Check sheet for the modelled part. Datum: model origin and axes. Units: mm. Face numbers are marked on the shaded views. A direction names the side the tool comes from. Round coordinates to 2 decimals unless told otherwise and drop trailing zeros. Order: outer loops, then holes, each group sorted by start corner. A loop starts at its lowest first (then second) coordinate and runs counter-clockwise, first axis right, second up. Notation, with made-up numbers: (66.25, 49) -> (107.25, 49) arc R21 ccw to (107.25, 72) -> close; hole circle Ø3 at (64.25, 88.25). An arc over 180 degrees is marked (long way). Answer in a Markdown table with one row per item.
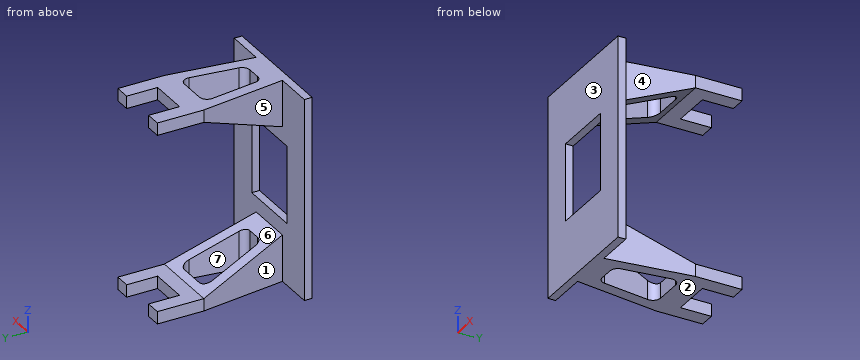
Autodesk Fusion 360 part; units mm, degrees
sketch "Esquisse1" plane through (0, 0, 0) normal (0, 0, 1) x (1, 0, 0)
  line L0 (27.5, 70) -> (52.5, 70)
  line L1 (52.5, 70) -> (52.5, 90)
  line L2 (27.5, 70) -> (27.5, 90)
  line L3 (27.5, 90) -> (17.5, 90)
  line L4 (52.5, 90) -> (62.5, 90)
  line L5 (62.5, 90) -> (62.5, 60)
  line L6 (17.5, 90) -> (17.5, 60)
  line L7 (17.5, 60) -> (25, 5)
  line L8 (25, 5) -> (0, 5)
  line L9 (0, 5) -> (0, 0)
  line L10 (0, 0) -> (80, 0)
  line L11 (80, 0) -> (80, 5)
  line L12 (80, 5) -> (55, 5)
  line L13 (55, 5) -> (62.5, 60)
  dimension "d1" = 70
  dimension "d2" = 25
  dimension "d3" = 20
  dimension "d4" = 10
  dimension "d5" = 30
  dimension "d8" = 5
  dimension "d10" = 10
  dimension "d27" = 80
  dimension "d28" = 45
  dimension "d29" = 17.5
  dimension "d30" = 30
extrude "Extrusion1" add sketch "Esquisse1" along normal blind 130
sketch "Esquisse2" plane through (62.5, 0, 0) normal (1, 0, 0) x (0, 0, -1)
  line L0 (0, 60) -> (0, 90)
  line L1 (0, 90) -> (-130, 90)
  line L2 (-130, 90) -> (-130, 60)
  line L3 (-130, 60) -> (0, 60)
  line L4 (-65, 90) -> (-65, -26) construction
  line L5 (-122, 90) -> (-122, 60)
  line L6 (-122, 60) -> (-100, 5)
  line L7 (-8, 90) -> (-8, 60)
  line L8 (-8, 60) -> (-30, 5)
  line L9 (-100, 5) -> (-30, 5)
  point P0 (-130, 5)
  point P1 (0, 5)
  dimension "d13" = 8
  dimension "d14" = 30
  dimension "d15" = 30
  dimension "d16" = 8
extrude "Extrusion2" cut sketch "Esquisse2" against normal blind 60 contours L3 L6 L8 L9 | L1 L3 L5 L7
sketch "Esquisse3" plane through (0, 0, 130) normal (0, 0, 1) x (1, 0, 0)
  line L0 (27.5, 70) -> (27.5, 90)
  line L1 (27.5, 90) -> (17.5, 90)
  line L2 (17.5, 90) -> (17.5, 60)
  line L3 (17.5, 60) -> (25, 5)
  line L4 (25, 5) -> (0, 5)
  line L5 (0, 5) -> (0, 0)
  line L6 (0, 0) -> (80, 0)
  line L7 (80, 0) -> (80, 5)
  line L8 (80, 5) -> (55, 5)
  line L9 (55, 5) -> (62.5, 60)
  line L10 (62.5, 60) -> (62.5, 90)
  line L11 (62.5, 90) -> (52.5, 90)
  line L12 (52.5, 90) -> (52.5, 70)
  line L13 (52.5, 70) -> (27.5, 70)
  line L14 (26.5252, 49.3244) -> (30.6161, 19.3244)
  line L15 (35.5702, 15) -> (44.4298, 15)
  line L16 (49.3839, 19.3244) -> (53.4748, 49.3244)
  line L17 (48.5207, 55) -> (31.4793, 55)
  arc A0 (31.4793, 55) -> (26.5252, 49.3244) centre (31.4793, 50) ccw
  arc A1 (53.4748, 49.3244) -> (48.5207, 55) centre (48.5207, 50) ccw
  arc A2 (30.6161, 19.3244) -> (35.5702, 15) centre (35.5702, 20) ccw
  arc A3 (44.4298, 15) -> (49.3839, 19.3244) centre (44.4298, 20) ccw
  dimension "d19" = 15
  dimension "d20" = 15
  dimension "d21" = 7.5
  dimension "d22" = 7.5
  dimension "d25" = 5
extrude "Extrusion3" cut sketch "Esquisse3" against normal blind 150 contours L14 L15 L16 L17 A0 A1 A2 A3
sketch "Esquisse4" plane through (0, 5, 0) normal (0, 1, 0) x (-1, 0, 0)
  line L0 (-55, 100) -> (-55, 130)
  line L1 (-55, 130) -> (-80, 130)
  line L2 (-80, 130) -> (-80, 0)
  line L3 (-80, 0) -> (-55, 0)
  line L4 (-55, 0) -> (-55, 30)
  line L5 (-55, 30) -> (-25, 30)
  line L6 (-25, 30) -> (-25, 0)
  line L7 (-25, 0) -> (0, 0)
  line L8 (0, 0) -> (0, 130)
  line L9 (0, 130) -> (-25, 130)
  line L10 (-25, 130) -> (-25, 100)
  line L11 (-25, 100) -> (-55, 100)
  line L12 (-60, 90) -> (-20, 90)
  line L13 (-20, 90) -> (-20, 40)
  line L14 (-20, 40) -> (-60, 40)
  line L15 (-60, 40) -> (-60, 90)
extrude "Extrusion4" cut sketch "Esquisse4" against normal blind 20 contours L12 L13 L14 L15
equation "d15 = d14"
equation "d16 = d13"
equation "d29 = ( d27 - d28 ) / 2"
Item 1: Mould release check, pull along Y, two halves, no side actions. Record for the marked faces 1, 2, 3 and 4: pulls with the +Y half, pulls with the -Y half, needs draft (parallel to the pull), parting line crosses it, or undercut.
Result sheet:
| item | result |
|---|---|
| face 1 | undercut |
| face 2 | needs draft |
| face 3 | pulls with the -Y half |
| face 4 | undercut |
Item 2: Depth check by flat-ended pin: P1, Ø4, axis at x = 38.5, z = 3, coming from the +Y side; P2, Ø3, axis at x = 13.5, z = 100.5, coming from the +Y side; P3, Ø12, axis at x = 49.5, z = 26.5, coming from the +Y side. Enter the tip coordinate at first touch or a pass-through.
Result sheet:
| item | result |
|---|---|
| P1 | stops at y = 70 |
| P2 | stops at y = 5 |
| P3 | stops at y = 28.48 |
Item 3: Cross-section at A-A (y = 76). Record the boundary of the cut face in (x, z), and give its area (3 significant figures).
Result sheet:
| item | result |
|---|---|
| outline | (17.5, 0) -> (27.5, 0) -> (27.5, 8) -> (17.5, 8) -> close; (17.5, 122) -> (27.5, 122) -> (27.5, 130) -> (17.5, 130) -> close; (52.5, 0) -> (62.5, 0) -> (62.5, 8) -> (52.5, 8) -> close; (52.5, 122) -> (62.5, 122) -> (62.5, 130) -> (52.5, 130) -> close |
| area | 320 mm^2 |
Item 4: Cross-section at D-D (y = 62). Record the boundary of the cut face in (x, z).
Result sheet:
| item | result |
|---|---|
| outline | (17.5, 0) -> (62.5, 0) -> (62.5, 8) -> (17.5, 8) -> close; (17.5, 122) -> (62.5, 122) -> (62.5, 130) -> (17.5, 130) -> close |
Item 5: Scan lines: line 1 (Z direction, x = 61.5, y = 71.5); line 2 (X direction, y = 22.5, z = 120); line 3 (Y direction, x = 76, z = 102). Record each from-to range of solid material in increasing order. Write a range as [from, to].
Result sheet:
| item | result |
|---|---|
| line 1 | z = [0, 8], [122, 130] |
| line 2 | x = [22.61, 30.18], [49.82, 57.39] |
| line 3 | y = [0, 5] |
Item 6: Cross-section at B-B (z = 63). Record the boundary of the cut face in (x, y).
Result sheet:
| item | result |
|---|---|
| outline | (0, 0) -> (20, 0) -> (20, 5) -> (0, 5) -> close; (60, 0) -> (80, 0) -> (80, 5) -> (60, 5) -> close |
Item 7: Set-up check for the marked faces 5, 6 and 7: record each of +Z, -Z, +X, -X, +Y, -Y from which the full face is reachable in a straight line by a thin tool's end or side.
Result sheet:
| item | result |
|---|---|
| face 5 | +Z, -Z, -X |
| face 6 | +X, -X, +Y |
| face 7 | +Z, -Z |
Item 8: Cross-section at C-C (x = 23.5). Record the boundary of the cut face in (y, z).
Result sheet:
| item | result |
|---|---|
| outline | (0, 0) -> (5, 0) -> (5, 40) -> (0, 40) -> close; (0, 90) -> (5, 90) -> (5, 130) -> (0, 130) -> close; (16, 0) -> (90, 0) -> (90, 8) -> (60, 8) -> (16, 25.6) -> close; (16, 104.4) -> (60, 122) -> (90, 122) -> (90, 130) -> (16, 130) -> close |
